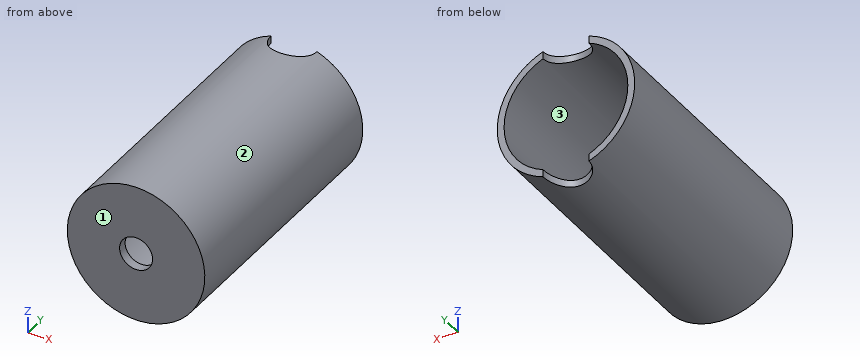
```python
from build123d import *

# Parameters (mm, degrees)
SKETCH1_R           = 15
SKETCH1_R_2         = 13.5
SKETCH1_R_3         = 3.6
BOSS_EXTRUDE1_DEPTH = 2
SKETCH1_3_R         = 15
SKETCH1_3_R_2       = 13.5
BOSS_EXTRUDE2_DEPTH = 57
SKETCH3_R           = 5
CUT_EXTRUDE2_DEPTH  = 57


with BuildPart() as part:
    # Sketch1 → Boss-Extrude1 (new body)
    # profile 1 of 2: a face of its own
    with BuildSketch(Plane(origin=(0, 0, 0), x_dir=(1, 0, 0), z_dir=(0, 1, 0))):
        with Locations(Location((0, 0, 0), (0, 0, 270))):
            Circle(SKETCH1_R)
        Circle(SKETCH1_R_2, mode=Mode.SUBTRACT)
    # profile 2 of 2: a face of its own
    with BuildSketch(Plane(origin=(0, 0, 0), x_dir=(1, 0, 0), z_dir=(0, 1, 0))):
        Circle(SKETCH1_R_2)
        with Locations(Location((0, 0, 0), (0, 0, 270))):
            Circle(SKETCH1_R_3, mode=Mode.SUBTRACT)
    extrude(amount=BOSS_EXTRUDE1_DEPTH)

    # Sketch1_3 → Boss-Extrude2 (add)
    with BuildSketch(Plane(origin=(0, 0, 0), x_dir=(1, 0, 0), z_dir=(0, 1, 0))):
        with Locations(Location((0, 0, 0), (0, 0, 270))):
            Circle(SKETCH1_3_R)
        with Locations(Location((0, 0, 0), (0, 0, 90))):
            Circle(SKETCH1_3_R_2, mode=Mode.SUBTRACT)
    extrude(amount=BOSS_EXTRUDE2_DEPTH)

    # Sketch3 → Cut-Extrude2 (cut)
    with BuildSketch(Plane.XY.offset(15)):
        with Locations((0, 57)):
            Circle(SKETCH3_R)
    extrude(amount=-CUT_EXTRUDE2_DEPTH, mode=Mode.SUBTRACT)


solid = part.part
```
Here's how the part is built. I have some questions about the finished solid (model axes, mm). Face numbers are marked on the shaded views. Round coordinates to 2 decimals unless told otherwise and drop trailing zeros. Write each loop counter-clockwise with the first axis right and the second up, starting at its lowest first coordinate (ties: lowest second). Pieces come first, ordered by that corner, then holes.
Q1. Will these pins go through, and if not, where does the flat tip stop? P1, Ø5, axis at x = 9.5, y = 24.5, coming from the -Z side; P2, Ø9.5, axis at x = 0, z = 0, coming from the +Y side; P3, Ø3, axis at x = 6.5, y = 48.5, coming from the -Z side; P4, Ø1.5, axis at x = 0.5, z = 12, coming from the -Y side.
Q2. If we section it at D-D on y = 13: Write out the boundary of the cut face in (x, z).
Q3. If we mould it in two halves opening along Z, with no side actions, what happens to the marked faces 1, 2 and 3? For each: +Z half, -Z half, draft (parallel to the pull), parting line (faces both ways), or undercut.
Q4. Please list where these lines run through material, in increasing order: probe 1 along X at (y, z) = (37, 0); probe 2 along X at (y, z) = (0.4, 0); probe 3 along Z at (x, y) = (-5, 5).
Q5. If we section it at A-A on x = 0: Write out the boundary of the cut face in (y, z), plus the area to 3 significant figures.
Q6. If we section it at C-C on z = 5: Write out the boundary of the cut face in (x, y), plus the area to 3 significant figures.
Q7. If we section it at B-B on z = 0: Write out the boundary of the cut face in (x, y).
Answer below:
1. P1: stops at z = -13.27
1. P2: stops at y = 2
1. P3: stops at z = -14.14
1. P4: stops at y = 0
2. outline: circle Ø30 at (0, 0); hole circle Ø27 at (0, 0)
3. face 1: draft
3. face 2: parting line
3. face 3: undercut
4. probe 1: x = -15 to -13.5, 13.5 to 15
4. probe 2: x = -15 to -3.6, 3.6 to 15
4. probe 3: z = -14.14 to -12.54, 12.54 to 14.14
5. outline: (0, -15) - (52, -15) - (52, -13.5) - (2, -13.5) - (2, -3.6) - (0, -3.6) - close; (0, 3.6) - (2, 3.6) - (2, 13.5) - (52, 13.5) - (52, 15) - (0, 15) - close
5. area: 196 mm2
6. outline: (-14.14, 0) - (14.14, 0) - (14.14, 57) - (12.54, 57) - (12.54, 2) - (-12.54, 2) - (-12.54, 57) - (-14.14, 57) - close
6. area: 233 mm2
7. outline: (-15, 0) - (-3.6, 0) - (-3.6, 2) - (-13.5, 2) - (-13.5, 57) - (-15, 57) - close; (3.6, 0) - (15, 0) - (15, 57) - (13.5, 57) - (13.5, 2) - (3.6, 2) - close
